Work out the finished part from the listing and answer in its coordinate system (mm). A direction names the side the tool comes from. Coordinates: 2 decimals unless noted, no trailing zeros. Loops run counter-clockwise (first coordinate to the right, second up) from the corner with the lowest first, then second, coordinate; pieces in that order, holes last. Notation, with made-up numbers: (-25, 18) -> (-2, 18) arc R17 ccw to (-2, 26) -> close; hole circle Ø11 at (51, 8). An arc over 180 degrees is marked (long way). Answer as CSV lines item,"result".
```python
from build123d import *

# Parameters (mm, degrees)
F0_R      = 31.5
F1_DEPTH  = 1.5
F3_DEPTH  = 3.5
F4_W      = 3.5
F4_H      = 3.5
F5_DEPTH  = 30
F6_R      = 0.75
F7_DEPTH  = 23
F8_R      = 0.75
F9_DEPTH  = 23
F10_R     = 0.925
F11_DEPTH = 2
F12_R     = 0.925
F13_DEPTH = 2
F6_R_2    = 0.925
F14_DEPTH = 2
F6_R_3    = 1.5625
F15_DEPTH = 0.35
F17_DEPTH = 0.75


with BuildPart() as f1:
    # F0 (on Top) → F1 (new body)
    with BuildSketch(Plane.XY):
        Circle(F0_R)
    extrude(amount=F1_DEPTH)

    # F2 (on Top) → F3 (join)
    with BuildSketch(Plane.XY):
        Polygon((-6.834524, 16.5), (-16.5, 6.834524), (-16.5, -6.834524), (-6.834524, -16.5), (6.834524, -16.5), (16.5, -6.834524), (16.5, 6.834524), (6.834524, 16.5), align=None)
        Polygon((6.213203, -15), (-6.213203, -15), (-15, -6.213203), (-15, 6.213203), (-6.213203, 15), (6.213203, 15), (15, 6.213203), (15, -6.213203), align=None, mode=Mode.SUBTRACT)
    extrude(amount=-F3_DEPTH)

    # F4 (on Top) → F5 (join)
    with BuildSketch(Plane.XY):
        with Locations((0, -13.25)):
            Rectangle(F4_W, F4_H)
        with Locations((13.25, 0)):
            Rectangle(F4_W, F4_H)
        with Locations((0, 13.25)):
            Rectangle(F4_W, F4_H)
        with Locations((-13.25, 0)):
            Rectangle(F4_W, F4_H)
    extrude(amount=-F5_DEPTH)

    # F6 (on face) → F7 (join, through all)
    with BuildSketch(Plane.XZ.offset(-11.5)):
        with Locations((0, -11)):
            Circle(F6_R)
        with Locations((0, -24)):
            Circle(F6_R)
    extrude(amount=F7_DEPTH)

    # F8 (on face) → F9 (join, through all)
    with BuildSketch(Plane(origin=(11.5, 0, 0), x_dir=(0, -1, 0), z_dir=(-1, 0, 0))):
        with Locations((0, -24)):
            Circle(F8_R)
        with Locations((0, -11)):
            Circle(F8_R)
    extrude(amount=F9_DEPTH)

    # F10 (on Front) → F11 (join, symmetric)
    with BuildSketch(Plane.XZ):
        with Locations((0, -11)):
            Circle(F10_R)
        with Locations((0, -24)):
            Circle(F10_R)
    extrude(amount=F11_DEPTH, both=True)

    # F12 (on Right) → F13 (join, symmetric)
    with BuildSketch(Plane.YZ):
        with Locations((0, -24)):
            Circle(F12_R)
        with Locations((0, -11)):
            Circle(F12_R)
    extrude(amount=F13_DEPTH, both=True)

    # F6 (on face) → F14 (join)
    with BuildSketch(Plane.XZ.offset(-11.5)):
        with Locations((0, -24)):
            Circle(F6_R_2)
        with Locations((0, -24)):
            Circle(F6_R, mode=Mode.SUBTRACT)
        with Locations((0, -11)):
            Circle(F6_R_2)
        with Locations((0, -11)):
            Circle(F6_R, mode=Mode.SUBTRACT)
    extrude(amount=F14_DEPTH)

    # F6 (on face) → F15 (join)
    with BuildSketch(Plane.XZ.offset(-11.5)):
        with Locations((0, -24)):
            Circle(F6_R_3)
        with Locations((0, -24)):
            Circle(F6_R_2, mode=Mode.SUBTRACT)
        with Locations((0, -11)):
            Circle(F6_R_3)
        with Locations((0, -11)):
            Circle(F6_R_2, mode=Mode.SUBTRACT)
    extrude(amount=F15_DEPTH)

    # F16 (on face) → F17 (join)
    with BuildSketch(Plane(origin=(0, 0, 0), x_dir=(1, 0, 0), z_dir=(0, 0, -1))):
        Polygon((9.722718, 13.611806), (13.611806, 9.722718), (22.097087, 18.208), (18.208, 22.097087), align=None)
        Polygon((-19.975767, 18.208), (-11.490485, 9.722718), (-7.601398, 13.611806), (-16.086679, 22.097087), align=None)
        Polygon((-16.086679, -19.975767), (-7.601398, -11.490485), (-11.490485, -7.601398), (-19.975767, -16.086679), align=None)
        Polygon((22.097087, -16.086679), (13.611806, -7.601398), (9.722718, -11.490485), (18.208, -19.975767), align=None)
    extrude(amount=F17_DEPTH)


solid = f1.part
```
(1) Consider line 1 along Y through (x, z) = (-5, -2); line 2 along Z through (x, y) = (5.5, -11.5); line 3 along Z through (x, y) = (0, 16). Determine where each line is inside the solid, lowest interval first.
Computed values:
line 1,"-16.5 to -15, 15 to 16.5"
line 2,"0 to 1.5"
line 3,"-3.5 to 1.5"
(2) For a pull along Y with two mould halves and no side action, classify faces 4 (the face through (-4, -15, -2)), 5 (the face through (-0.924, -1.208, -10.959)), 6 (the face through (-18.004, -20.18, -0.37)), 7 (the face through (0, -13, -30)) as pulls with the +Y half, pulls with the -Y half, needs draft (parallel to the pull), parting line crosses it, or undercut.
Computed values:
face 4,"undercut"
face 5,"undercut"
face 6,"pulls with the -Y half"
face 7,"needs draft"
(3) A cutting plane is placed at B-B, the plane y = -3. Write down the section's boundary in (x, z).
Computed values:
outline,"(-31.36, 0) -> (-16.5, 0) -> (-16.5, -3.5) -> (-15, -3.5) -> (-15, 0) -> (15, 0) -> (15, -3.5) -> (16.5, -3.5) -> (16.5, 0) -> (31.36, 0) -> (31.36, 1.5) -> (-31.36, 1.5) -> close; circle Ø1.5 at (0, -24); circle Ø1.5 at (0, -11)"
(4) Which of the six approach directions +Z, -Z, +X, -X, +Y, -Y give full straight-line access (tool end or side, diameter ignored) to faces 1 (the face through (6.816, 0.163, -24.732)), 2 (the face through (-15, 4, -2)), 3 (the face through (-15, 15, -0.75))?
Computed values:
face 1,"none"
face 2,"-Z"
face 3,"-Z, -X, +Y"
(5) A cutting plane is placed at D-D, the plane y = 21. Write down the section's boundary in (x, z).
Computed values:
outline,"(-23.48, 0) -> (23.48, 0) -> (23.48, 1.5) -> (-23.48, 1.5) -> close"
(6) A cutting plane is placed at A-A, the plane z = -19.5. Write down the section's boundary in (x, y).
Computed values:
outline,"(-15, -1.75) -> (-11.5, -1.75) -> (-11.5, 1.75) -> (-15, 1.75) -> close; (-1.75, -15) -> (1.75, -15) -> (1.75, -11.5) -> (-1.75, -11.5) -> close; (-1.75, 11.5) -> (1.75, 11.5) -> (1.75, 15) -> (-1.75, 15) -> close; (11.5, -1.75) -> (15, -1.75) -> (15, 1.75) -> (11.5, 1.75) -> close"
(7) A cutting plane is placed at C-C, the plane x = 12.5. Write down the section's boundary in (y, z), and give its area (3 significant figures).
Computed values:
outline,"(-28.91, 0) -> (-16.39, 0) -> (-16.39, -0.75) -> (-10.83, -0.75) -> (-10.83, -3.5) -> (-8.71, -3.5) -> (-8.71, 0) -> (-1.75, 0) -> (-1.75, -30) -> (1.75, -30) -> (1.75, 0) -> (8.71, 0) -> (8.71, -3.5) -> (10.83, -3.5) -> (10.83, -0.75) -> (14.27, -0.75) -> (14.27, 0) -> (28.91, 0) -> (28.91, 1.5) -> (-28.91, 1.5) -> close"
area,"213 mm2"
(8) Flat-ended cylindrical pins translate along their axes: pin 1 Ø0.9 at (x, z) = (0.5, -11) entering from -Y; pin 2 Ø3 at (x, z) = (-14, -14) entering from -Y; pin 3 Ø4 at (y, z) = (17.5, -25) entering from +X; pin 4 Ø3 at (y, z) = (-3.5, -9) entering from +X. Find the tip coordinate at first contact, or state that the pin passes through.
Computed values:
pin 1,"y = -15"
pin 2,"y = -1.75"
pin 3,"through"
pin 4,"x = 0.56"
